```python
from build123d import *

# Parameters (mm, degrees)
SKETCH2_R          = 1.5
CUT_EXTRUDE1_DEPTH = 13.350354246


with BuildPart() as part:
    # Sketch1 → Revolve1 (revolve)
    with BuildSketch(Plane.YZ):
        Polygon((0, 0), (0, 5.125), (1.5, 5.125), (10, 4.275), (10, 3.875), (1.5, 3.875), (1.5, 0), align=None)
    revolve(axis=Axis((0, 1.5, 0), (0, -1, 0)))

    # Sketch2 → Cut-Extrude1 (cut, through all)
    with BuildSketch(Plane.XZ):
        with Locations(Location((0, 0, 0), (0, 0, 270))):
            Circle(SKETCH2_R)
    extrude(amount=-CUT_EXTRUDE1_DEPTH, mode=Mode.SUBTRACT)


solid = part.part
```
Here's how the part is built. I have some questions about the finished solid (model axes, mm). A direction names the side the tool comes from. Give positions to 0.01 mm unless a question says otherwise; leave off trailing zeros. Loops run counter-clockwise (first coordinate to the right, second up) from the corner with the lowest first, then second, coordinate; pieces in that order, holes last. Notation, with made-up numbers: M -13.75,82 L 12.25,82 A19 cw 12.25,102 Z; hole C 67,72.5 d4. An arc over 180 degrees is marked long. Put each result on its own line as item: value. Start each with the question number.
(1) Will these pins go through, and if not, where does the flat tip stop? pin 1 Ø3 at (y, z) = (9, -1.5) entering from +X; pin 2 Ø4.5 at (x, z) = (0, 0) entering from +Y; pin 3 Ø6 at (y, z) = (4.5, 1.5) entering from +X.
(2) If we mould it in two halves opening along Z, with no side actions, what happens to faces 1 (the cylindrical face through (5.003, 0.76, -1.111)), 2 (the cylindrical face through (-3.842, 5.69, -0.504)), 3 (the flat face through (-1, 10, -4))? For each: +Z half, -Z half, draft (parallel to the pull), parting line (faces both ways), or undercut.
(3) I want a section at C-C on y = 7.25. Please give me the cut outline in (x, z) (3 decimals), then the cut area to 3 significant figures.
(4) I want a section at B-B on z = 0. Please give me the cut outline in (x, y) (3 decimals), then the cut area to 3 significant figures.
(5) I want a section at D-D on y = 1. Please give me the cut outline in (x, z) (3 decimals), then the cut area to 3 significant figures.
(6) I want a section at A-A on x = 0. Please give me the cut outline in (y, z) (3 decimals), then the cut area to 3 significant figures.
(7) For faces 4 (the cylindrical face through (0.45, 0.74, -1.43)), 5 (the flat face through (2, 1.5, 0)), which set-ups out of +Z, -Z, +X, -X, +Y, -Y let a thin tool reach every point of the face, with its end or its side?
(8) I need wall thicknesses on line 1 along Y through (x, z) = (-0.25, -3.25); line 2 along X through (y, z) = (0.95, 0) (3 decimals); line 3 along Z through (x, y) = (-3.25, 9). Which ranges of each line are inside material? Lowest first, please. Write a range as [from, to].
Answer block:
1. pin 1: x = 4.46
1. pin 2: y = 1.5
1. pin 3: x = 5.09
2. face 1: parting line
2. face 2: undercut
2. face 3: draft
3. outline: C 0,0 d9.1; hole C 0,0 d7.75
3. area: 17.9 mm^2
4. outline: M -5.125,0 L -1.5,0 L -1.5,1.5 L -3.875,1.5 L -3.875,10 L -4.275,10 L -5.125,1.5 Z; M 1.5,0 L 5.125,0 L 5.125,1.5 L 4.275,10 L 3.875,10 L 3.875,1.5 L 1.5,1.5 Z
4. area: 24.9 mm^2
5. outline: C 0,0 d10.25; hole C 0,0 d3
5. area: 75.4 mm^2
6. outline: M 0,-5.125 L 1.5,-5.125 L 10,-4.275 L 10,-3.875 L 1.5,-3.875 L 1.5,-1.5 L 0,-1.5 Z; M 0,1.5 L 1.5,1.5 L 1.5,3.875 L 10,3.875 L 10,4.275 L 1.5,5.125 L 0,5.125 Z
6. area: 24.9 mm^2
7. face 4: +Y, -Y
7. face 5: +Y
8. line 1: [0, 1.5]
8. line 2: [-5.125, -1.5], [1.5, 5.125]
8. line 3: [-2.93, -2.11], [2.11, 2.93]
